Geometry check sheet. Reference: drawing and pictorial views, mm from the part's lowest x, y, z. Round coordinates to 2 decimals unless told otherwise and drop trailing zeros. Order: outer loops, then holes, each group sorted by start corner. A loop starts at its lowest first (then second) coordinate and runs counter-clockwise, first axis right, second up. Notation, with made-up numbers: (-8.75, 37.5) -> (20.25, 37.5) arc R15 cw to (20.25, 48.5) -> close; hole circle Ø7 at (68, -17.75). An arc over 180 degrees is marked (long way). Put each result on its own line as item: value.
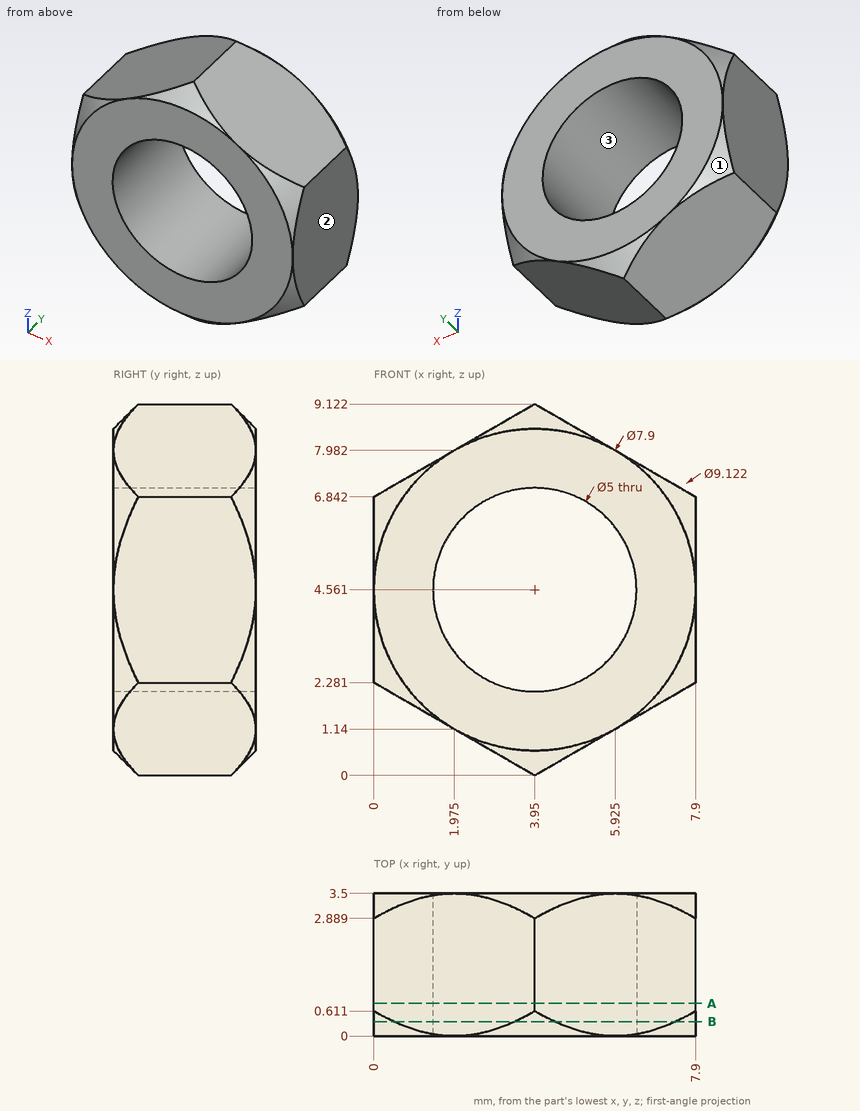
Item 1: Depth check by flat-ended pin: pin 1 Ø1.5 at (x, y) = (5, 2.5) entering from -Z. Enter the tip coordinate at first touch or a pass-through.
Geometry check:
pin 1: z = 0.17
Item 2: Sectioned sample at B-B, the plane y = 0.35. Record the boundary of the cut face in (x, z).
Geometry check:
outline: (0, 2.86) arc R4.3 ccw to (0.5, 1.99) -> (3.45, 0.29) arc R4.3 ccw to (4.45, 0.29) -> (7.4, 1.99) arc R4.3 ccw to (7.9, 2.86) -> (7.9, 6.26) arc R4.3 ccw to (7.4, 7.13) -> (4.45, 8.83) arc R4.3 ccw to (3.45, 8.83) -> (0.5, 7.13) arc R4.3 ccw to (0, 6.26) -> close; hole circle Ø5 at (3.95, 4.56)
Item 3: Sectioned sample at A-A, the plane y = 0.8. Record the boundary of the cut face in (x, z).
Geometry check:
outline: (0, 2.28) -> (3.95, 0) -> (7.9, 2.28) -> (7.9, 6.84) -> (3.95, 9.12) -> (0, 6.84) -> close; hole circle Ø5 at (3.95, 4.56)
Item 4: Release check for a two-part mould opening along X. For the marked faces 1, 2 and 3 record: pulls with the +X half, pulls with the -X half, needs draft (parallel to the pull), parting line crosses it, or undercut.
Geometry check:
face 1: pulls with the -X half
face 2: pulls with the +X half
face 3: undercut
Item 5: Material ranges on line 1 along Z through (x, y) = (2.5, 1.55) (1 decimal); line 2 along X through (y, z) = (0.2, 3.75) (1 decimal); line 3 along Z through (x, y) = (3.25, 1.2) (1 decimal), recorded low to high.
Geometry check:
line 1: 0.8 to 2.5, 6.6 to 8.3
line 2: 0 to 1.6, 6.3 to 7.9
line 3: 0.4 to 2.2, 7 to 8.7
